```python
from build123d import *

# Parameters (mm, degrees)
SKETCH_1_R                       = 39
EXTRUDE_1_DEPTH                  = 2.5
FILLET_1_R                       = 5
SKETCH_2_W                       = 8
SKETCH_2_H                       = 2.5
EXTRUDE_2_DEPTH                  = 5
SKETCH_3_W                       = 8
SKETCH_3_H                       = 2.5
EXTRUDE_3_DEPTH                  = 1
FILLET_4_R                       = 0.5
FILLET_5_R                       = 2
PATTERN_CIRCULAR_7_COUNT         = 4
FILLET_4_OF_PATTERN_CIRCULAR_7_R = 0.5
FILLET_5_OF_PATTERN_CIRCULAR_7_R = 2
CUT_EXTRUDE_1_DEPTH              = 56.380501984
PATTERN_CIRCULAR_8_COUNT         = 4


# Some blends are built 0.0001 mm under size
with BuildPart() as part:
    # ｽｹｯﾁ1 → ﾎﾞｽ - 押し出し1 (new body)
    with BuildSketch(Plane.XY):
        Circle(SKETCH_1_R)
    extrude(amount=EXTRUDE_1_DEPTH)

    # ﾌｨﾚｯﾄ1
    # the kernel refuses this fillet: 5 mm, written as the material it takes off along each edge
    with BuildSketch(Plane(origin=(0, 0, 2.5), x_dir=(1, 0, 0), z_dir=(0, -1, 0))) as fillet_1_piece_1:
        with BuildLine():
            CenterArc((34.669872981, -5), FILLET_1_R, 30, 60)
            Line((34.669872981, 0), (34.669872981, 0.1))
            Line((34.669872981, 0.1), (39, 0.1))
            Line((39, 0.1), (39.1, 0))
            ThreePointArc((39.1, 0), (39.1, -1.25), (39.08660254, -2.45))
            Line((39.08660254, -2.45), (39, -2.5))
        make_face()
    revolve(axis=Axis((0, 0, 2.5), (0, 0, 1)), mode=Mode.SUBTRACT)

    # ｽｹｯﾁ2 → ﾎﾞｽ - 押し出し2 (add)
    with BuildSketch(Plane(origin=(0, 0, 0), x_dir=(-1, 0, 0), z_dir=(0, 0, -1))):
        with Locations((0, 35)):
            Rectangle(SKETCH_2_W, SKETCH_2_H)
    extrude_2 = extrude(amount=EXTRUDE_2_DEPTH)

    # ｽｹｯﾁ3 → ﾎﾞｽ - 押し出し3 (add)
    with BuildSketch(Plane(origin=(0, 36.25, 0), x_dir=(1, 0, 0), z_dir=(0, 1, 0))):
        with Locations((0, 3.75)):
            Rectangle(SKETCH_3_W, SKETCH_3_H)
    extrude_3 = extrude(amount=EXTRUDE_3_DEPTH)

    # ﾌｨﾚｯﾄ4
    fillet_4_edges = [part.edges().sort_by_distance(p)[0] for p in [
        (0, 37.25, -2.5),
    ]]
    fillet(fillet_4_edges, radius=FILLET_4_R)

    # ﾌｨﾚｯﾄ5
    fillet_5_edges = [part.edges().sort_by_distance(p)[0] for p in [
        (0, 37.25, -5),
    ]]
    fillet(fillet_5_edges, radius=FILLET_5_R - 0.0001)  # a hair under: the kernel refuses the full size

    # 円形ﾊﾟﾀｰﾝ7: ﾎﾞｽ - 押し出し2, ﾎﾞｽ - 押し出し3 ×4 about axis
    pattern_circular_7_axis = Axis((0, 0, 0), (0, 0, 1))
    add([extrude_2.rotate(pattern_circular_7_axis, i * 360 / PATTERN_CIRCULAR_7_COUNT) for i in range(1, PATTERN_CIRCULAR_7_COUNT)])
    add([extrude_3.rotate(pattern_circular_7_axis, i * 360 / PATTERN_CIRCULAR_7_COUNT) for i in range(1, PATTERN_CIRCULAR_7_COUNT)])

    # ﾌｨﾚｯﾄ4 of 円形ﾊﾟﾀｰﾝ7
    fillet_4_of_pattern_circular_7_edges = [part.edges().sort_by_distance(p)[0] for p in [
        (-37.25, 0, -2.5),
        (0, -37.25, -2.5),
        (37.25, 0, -2.5),
    ]]
    fillet(fillet_4_of_pattern_circular_7_edges, radius=FILLET_4_OF_PATTERN_CIRCULAR_7_R)

    # ﾌｨﾚｯﾄ5 of 円形ﾊﾟﾀｰﾝ7
    fillet_5_of_pattern_circular_7_edges = [part.edges().sort_by_distance(p)[0] for p in [
        (-37.25, 0, -5),
        (0, -37.25, -5),
        (37.25, 0, -5),
    ]]
    fillet(fillet_5_of_pattern_circular_7_edges, radius=FILLET_5_OF_PATTERN_CIRCULAR_7_R - 0.0001)  # a hair under: the kernel refuses the full size

    # ｽｹｯﾁ7 → ｶｯﾄ - 押し出し1 (cut, through all)
    with BuildSketch(Plane(origin=(0, 0, 0), x_dir=(-1, 0, 0), z_dir=(0, 0, -1))):
        with BuildLine():
            Line((24.677925359, 4), (33.763886032, 4))
            ThreePointArc((33.763886032, 4), (24.04163056, 24.04163056), (4, 33.763886032))
            Line((4, 33.763886032), (4, 24.677925359))
            ThreePointArc((4, 24.677925359), (17.67766953, 17.67766953), (24.677925359, 4))
        make_face()
    cut_extrude_1 = extrude(amount=-CUT_EXTRUDE_1_DEPTH, mode=Mode.SUBTRACT)

    # 円形ﾊﾟﾀｰﾝ8: ｶｯﾄ - 押し出し1 ×4 about axis
    pattern_circular_8_axis = Axis((0, 0, 0), (0, 0, -1))
    for i in range(1, PATTERN_CIRCULAR_8_COUNT):
        add(cut_extrude_1.rotate(pattern_circular_8_axis, i * 360 / PATTERN_CIRCULAR_8_COUNT), mode=Mode.SUBTRACT)


solid = part.part
```
The listing builds one solid part. Answer for the finished solid, in the listing's coordinates (mm). A direction names the side the tool comes from. Give positions to 0.01 mm unless a question says otherwise; leave off trailing zeros. Loops run counter-clockwise (first coordinate to the right, second up) from the corner with the lowest first, then second, coordinate; pieces in that order, holes last. Notation, with made-up numbers: M 0.5,88.5 L 25.5,88.5 A6 ccw 25.5,97.5 Z; hole C 25,31.5 d10. An arc over 180 degrees is marked long. One line per item, written item: value.
1. Each of these flat-tipped pins is pushed along its axis until it touches: P1, Ø8, axis at x = -20, y = 17, coming from the +Z side; P2, Ø1, axis at x = -25.5, z = 1.5, coming from the -Y side; P3, Ø2, axis at y = -28.5, z = 0.5, coming from the -X side; P4, Ø4, axis at x = 4, y = 16.5, coming from the -Z side. Where does it stop, or does it pass through?
Found:
P1: z = 2.5
P2: y = -28.63
P3: x = -27.52
P4: z = 0
2. Find the intervals of material crossed by probe 1 along X at (y, z) = (-4.5, 0.75); probe 2 along Y at (x, z) = (9.5, 1.5); probe 3 along X at (y, z) = (-29.5, 0.5), in increasing order.
Found:
probe 1: -38.21 to -33.7, -24.59 to 24.59, 33.7 to 38.21
probe 2: -36.45 to -32.65, -23.12 to 23.12, 32.65 to 36.45
probe 3: -25 to -16.9, -4 to 4, 16.9 to 25
3. Section A-A on z = -1.5 is taken. Determine the outline of the cut face in (x, y), plus the area to 3 significant figures.
Found:
outline: M -36.25,-4 L -33.75,-4 L -33.75,4 L -36.25,4 Z; M -4,-36.25 L 4,-36.25 L 4,-33.75 L -4,-33.75 Z; M -4,33.75 L 4,33.75 L 4,36.25 L -4,36.25 Z; M 33.75,-4 L 36.25,-4 L 36.25,4 L 33.75,4 Z
area: 80.0 mm^2
4. Section B-B on x = 26 is taken. State how many separate pieces and enclosed holes the cut face has, plus the area to 3 significant figures.
Found:
separate pieces: 3
enclosed holes: 0
area: 47.2 mm^2
5. For faces 4 (the face through (0, 36.25, -1)), 5 (the face through (-23.816, -24.265, 1.232)), 6 (the face through (-4, -30.9, 0.5)), determine the directions among +Z, -Z, +X, -X, +Y, -Y from which every point of the face is accessible in a straight line to the end or side of a thin tool.
Found:
face 4: +X, -X, +Y
face 5: +Z, -Z
face 6: -Z
6. For a pull along Y with two mould halves and no side action, classify faces 1 (the face through (-36.68, 0.06, -4.4)), 2 (the face through (0.06, 36.68, -4.4)), 3 (the face through (4, 30.9, 0.5)) as pulls with the +Y half, pulls with the -Y half, needs draft (parallel to the pull), parting line crosses it, or undercut.
Found:
face 1: needs draft
face 2: pulls with the +Y half
face 3: undercut
